Check sheet for the modelled part. Datum: model origin and axes. Units: mm. Coordinates: 2 decimals unless noted, no trailing zeros. Write each loop counter-clockwise with the first axis right and the second up, starting at its lowest first coordinate (ties: lowest second). Pieces come first, ordered by that corner, then holes. Notation, with made-up numbers: (-39, -23.75) -> (-4, -23.75) arc R33 cw to (-4, 15.25) -> close; hole circle Ø5 at (9.5, 5.25). An arc over 180 degrees is marked (long way). One line per item, written item: value. Start each with the question number.
1) Gauge pin test, flat end, axial feed: P1, Ø2.5, axis at x = 17.5, z = -16.7, coming from the +Y side. Record the tip position at first contact, or that the pin passes through.
2) Sectioned sample at B-B on x = 17.5. Enter the section's corners in (y, z), plus the area to 3 significant figures.
3) Sectioned sample at A-A on z = -16.7. Enter the section's corners in (x, y).
4) Scan lines: line 1 along X through (y, z) = (0.1, -16.7); line 2 along Z through (x, y) = (-17.5, 0.35); line 3 along Z through (x, y) = (-17.5, 0.6). Record each from-to range of solid material in increasing order. Write a range as [from, to].
5) Draft check along X on faces 1 (the cylindrical face through (17.43, 0.28, -18.4)), 2 (the flat face through (-22.5, 1, 0)), 3 (the flat face through (0, 0, 0)). Enter one of: +X half, -X half, draft (parallel to the pull), parting line (faces both ways), or undercut.
6) Sectioned sample at C-C on y = 1.3. Enter the section's corners in (x, z), plus the area to 3 significant figures.
```python
from build123d import *

# Parameters (mm, degrees)
SKETCH1_W                                      = 45
SKETCH1_H                                      = 55
SKETCH1_W_2                                    = 5
SKETCH1_H_2                                    = 2
BOSS_EXTRUDE1_DEPTH                            = 2
CSK_FOR_M3_FLAT_HEAD_MACHINE_SCREW1_AT_2_COUNT = 2
CSK_FOR_M3_FLAT_HEAD_MACHINE_SCREW1_AT_2_PITCH = 35
CSK_FOR_M3_FLAT_HEAD_MACHINE_SCREW1_AT_3_COUNT = 2
CSK_FOR_M3_FLAT_HEAD_MACHINE_SCREW1_AT_3_PITCH = 48.379334431
CSK_FOR_M3_FLAT_HEAD_MACHINE_SCREW1_AT_4_COUNT = 2
CSK_FOR_M3_FLAT_HEAD_MACHINE_SCREW1_AT_4_PITCH = 33.4


with BuildPart() as part:
    # Sketch1 → Boss-Extrude1 (new body)
    # profile 1 of 3: a face of its own
    with BuildSketch(Plane(origin=(0, 0, 0), x_dir=(1, 0, 0), z_dir=(0, 1, 0))):
        Rectangle(SKETCH1_W, SKETCH1_H)
        with Locations((0, 26.25)):
            Rectangle(SKETCH1_W_2, SKETCH1_H_2, mode=Mode.SUBTRACT)
        with Locations((0, -26.25)):
            Rectangle(SKETCH1_W_2, SKETCH1_H_2, mode=Mode.SUBTRACT)
    # profile 2 of 3: a face of its own
    with BuildSketch(Plane(origin=(0, 0, 0), x_dir=(1, 0, 0), z_dir=(0, 1, 0))):
        with Locations((0, 26.25)):
            Rectangle(SKETCH1_W_2, SKETCH1_H_2)
    # profile 3 of 3: a face of its own
    with BuildSketch(Plane(origin=(0, 0, 0), x_dir=(1, 0, 0), z_dir=(0, 1, 0))):
        with Locations((0, -26.25)):
            Rectangle(SKETCH1_W_2, SKETCH1_H_2)
    extrude(amount=BOSS_EXTRUDE1_DEPTH)

    # Sketch5 → CSK for M3 Flat Head Machine Screw1 (revolve, cut)
    with BuildSketch(Plane(origin=(-17.5, 2, -16.7), x_dir=(0, 0, 1), z_dir=(1, 0, 0))):
        Polygon((0, 0), (0, 2), (1.7, 2), (1.7, 1.45), (3.15, 0), align=None)
    csk_for_m3_flat_head_machine_screw1 = revolve(axis=Axis((-17.5, 8.35, -16.7), (0, -1, 0)), mode=Mode.SUBTRACT)

    # CSK for M3 Flat Head Machine Screw1 at 2: CSK for M3 Flat Head Machine Screw1 ×2
    with Locations(*[(i * CSK_FOR_M3_FLAT_HEAD_MACHINE_SCREW1_AT_2_PITCH, 0, 0) for i in range(1, CSK_FOR_M3_FLAT_HEAD_MACHINE_SCREW1_AT_2_COUNT)]):
        add(csk_for_m3_flat_head_machine_screw1, mode=Mode.SUBTRACT)

    # CSK for M3 Flat Head Machine Screw1 at 3: CSK for M3 Flat Head Machine Screw1 ×2
    with Locations(*[Vector(0.7234493903552432, 0, 0.6903774182247178) * (i * CSK_FOR_M3_FLAT_HEAD_MACHINE_SCREW1_AT_3_PITCH) for i in range(1, CSK_FOR_M3_FLAT_HEAD_MACHINE_SCREW1_AT_3_COUNT)]):
        add(csk_for_m3_flat_head_machine_screw1, mode=Mode.SUBTRACT)

    # CSK for M3 Flat Head Machine Screw1 at 4: CSK for M3 Flat Head Machine Screw1 ×2
    with Locations(*[(0, 0, i * CSK_FOR_M3_FLAT_HEAD_MACHINE_SCREW1_AT_4_PITCH) for i in range(1, CSK_FOR_M3_FLAT_HEAD_MACHINE_SCREW1_AT_4_COUNT)]):
        add(csk_for_m3_flat_head_machine_screw1, mode=Mode.SUBTRACT)


solid = part.part
```
Answers:
1. P1: passes through
2. outline: (0, -27.5) -> (2, -27.5) -> (2, -19.85) -> (0.55, -18.4) -> (0, -18.4) -> close; (0, -15) -> (0.55, -15) -> (2, -13.55) -> (2, 13.55) -> (0.55, 15) -> (0, 15) -> close; (0, 18.4) -> (0.55, 18.4) -> (2, 19.85) -> (2, 27.5) -> (0, 27.5) -> close
2. area: 92.2 mm2
3. outline: (-22.5, 0) -> (-19.2, 0) -> (-19.2, 0.55) -> (-20.65, 2) -> (-22.5, 2) -> close; (-15.8, 0) -> (15.8, 0) -> (15.8, 0.55) -> (14.35, 2) -> (-14.35, 2) -> (-15.8, 0.55) -> close; (19.2, 0) -> (22.5, 0) -> (22.5, 2) -> (20.65, 2) -> (19.2, 0.55) -> close
4. line 1: x = [-22.5, -19.2], [-15.8, 15.8], [19.2, 22.5]
4. line 2: z = [-27.5, -18.4], [-15, 15], [18.4, 27.5]
4. line 3: z = [-27.5, -18.45], [-14.95, 14.95], [18.45, 27.5]
5. face 1: undercut
5. face 2: -X half
5. face 3: draft
6. outline: (-22.5, -27.5) -> (22.5, -27.5) -> (22.5, 27.5) -> (-22.5, 27.5) -> close; hole circle Ø4.9 at (-17.5, -16.7); hole circle Ø4.9 at (-17.5, 16.7); hole circle Ø4.9 at (17.5, -16.7); hole circle Ø4.9 at (17.5, 16.7)
6. area: 2,400 mm2
